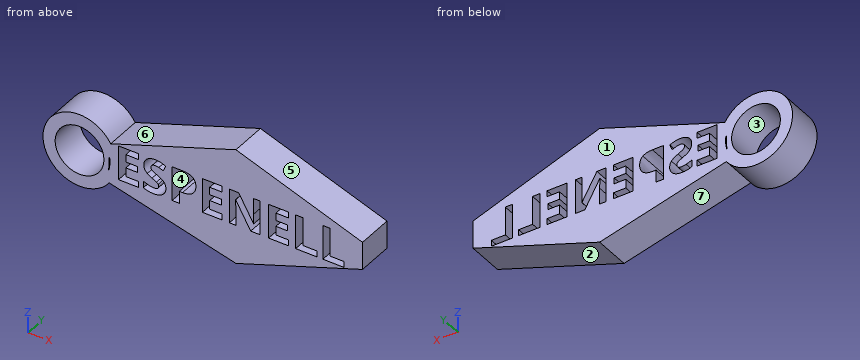
```python
from build123d import *

# Parameters (mm, degrees)
F0_R     = 10
F1_DEPTH = 15


with BuildPart() as f1:
    # F0 (on Front) → F1 (new body)
    with BuildSketch(Plane.XZ):
        with BuildLine():
            ThreePointArc((-51.9289774608, 2.6432993809), (-51.6588535234, -0.5600733653), (-52.2146643877, -3.726402182))
            Line((-52.2146643877, -3.726402182), (-52.2146643877, -8.726402182))
            Line((-52.2146643877, -8.726402182), (-51.9870151319, -8.7836093454))
            ThreePointArc((-51.9870151319, -8.7836093454), (-49.874136957, -4.6157733907), (-49.1462999327, 0))
            ThreePointArc((-49.1462999327, 0), (-49.7101962212, 4.0741759452), (-51.3594878837, 7.8420301978))
            Line((-51.3594878837, 7.8420301978), (-51.9289774608, 7.6432993809))
            Line((-51.9289774608, 7.6432993809), (-51.9289774608, 2.6432993809))
        make_face()
        with BuildLine():
            Line((-52.2146643877, -8.726402182), (-52.2146643877, -3.726402182))
            Line((-52.2146643877, -3.726402182), (-51.9289774608, 2.6432993809))
            Line((-51.9289774608, 2.6432993809), (-51.9289774608, 7.6432993809))
            Line((-51.9289774608, 7.6432993809), (-51.3594878837, 7.8420301978))
            ThreePointArc((-51.3594878837, 7.8420301978), (-79.1356264541, 0.565765353), (-51.9870151319, -8.7836093454))
            Line((-51.9870151319, -8.7836093454), (-52.2146643877, -8.726402182))
        make_face()
        with Locations((-64.1462999327, 0)):
            Circle(F0_R, mode=Mode.SUBTRACT)
        with BuildLine():
            ThreePointArc((-49.1462999327, 0), (-49.874136957, -4.6157733907), (-51.9870151319, -8.7836093454))
            Line((-51.9870151319, -8.7836093454), (0, -21.8476962826))
            Line((0, -21.8476962826), (51.9289774608, -3.726402182))
            Line((51.9289774608, -3.726402182), (51.9289774608, 7.6432993809))
            Line((51.9289774608, 7.6432993809), (0, 25.7645934815))
            Line((0, 25.7645934815), (-51.3594878837, 7.8420301978))
            ThreePointArc((-51.3594878837, 7.8420301978), (-49.7101962212, 4.0741759452), (-49.1462999327, 0))
        make_face()
        Polygon((-40.0178585444, -3.4319313488), (-40.0178585444, -5.9052360061), (-48.1519392362, -5.9052360061), (-48.1519392362, 8.2204252181), (-40.0178585444, 8.2204252181), (-40.0178585444, 5.7656703457), (-45.15614897, 5.7656703457), (-45.15614897, 2.6647646316), (-40.3733960889, 2.6647646316), (-40.3733960889, 0.2100097592), (-45.15614897, 0.2100097592), (-45.15614897, -3.4319313488), align=None, mode=Mode.SUBTRACT)
        with BuildLine():
            add(Edge.make_bspline(
                [(-29.4676683654, 0.3506789616), (-28.7334060453, -0.5999975161), (-28.7334060453, -1.9819564934)],
                knots=[0, 0, 0, 1, 1, 1], degree=2))
            add(Edge.make_bspline(
                [(-28.7334060453, -1.9819564934), (-28.7334060453, -3.895675972), (-30.1107275763, -4.9978423599)],
                knots=[0, 0, 0, 1, 1, 1], degree=2))
            add(Edge.make_bspline(
                [(-30.1107275763, -4.9978423599), (-31.4880491074, -6.1000087479), (-33.939712349, -6.1000087479)],
                knots=[0, 0, 0, 1, 1, 1], degree=2))
            add(Edge.make_bspline(
                [(-33.939712349, -6.1000087479), (-36.2027861105, -6.1000087479), (-37.9402826322, -5.2467186411)],
                knots=[0, 0, 0, 1, 1, 1], degree=2))
            Line((-37.9402826322, -5.2467186411), (-37.9402826322, -2.4642509016))
            add(Edge.make_bspline(
                [(-37.9402826322, -2.4642509016), (-36.5119491926, -3.1042184817), (-35.5210815143, -3.3639154707)],
                knots=[0, 0, 0, 1, 1, 1], degree=2))
            add(Edge.make_bspline(
                [(-35.5210815143, -3.3639154707), (-34.5302138359, -3.6236124597), (-33.7078400374, -3.6236124597)],
                knots=[0, 0, 0, 1, 1, 1], degree=2))
            add(Edge.make_bspline(
                [(-33.7078400374, -3.6236124597), (-32.7247014361, -3.6236124597), (-32.197578381, -3.2479793149)],
                knots=[0, 0, 0, 1, 1, 1], degree=2))
            add(Edge.make_bspline(
                [(-32.197578381, -3.2479793149), (-31.6704553259, -2.87234617), (-31.6704553259, -2.127263142)],
                knots=[0, 0, 0, 1, 1, 1], degree=2))
            add(Edge.make_bspline(
                [(-31.6704553259, -2.127263142), (-31.6704553259, -1.7129846119), (-31.9023276375, -1.3883633756)],
                knots=[0, 0, 0, 1, 1, 1], degree=2))
            add(Edge.make_bspline(
                [(-31.9023276375, -1.3883633756), (-32.1341999491, -1.0637421394), (-32.5840322337, -0.7653997651)],
                knots=[0, 0, 0, 1, 1, 1], degree=2))
            add(Edge.make_bspline(
                [(-32.5840322337, -0.7653997651), (-33.0338645182, -0.4670573908), (-34.4158234955, 0.1914599742)],
                knots=[0, 0, 0, 1, 1, 1], degree=2))
            add(Edge.make_bspline(
                [(-34.4158234955, 0.1914599742), (-35.708125179, 0.8005112461), (-36.3558218361, 1.3600964248)],
                knots=[0, 0, 0, 1, 1, 1], degree=2))
            add(Edge.make_bspline(
                [(-36.3558218361, 1.3600964248), (-37.0035184933, 1.9196816036), (-37.389972346, 2.6647646316)],
                knots=[0, 0, 0, 1, 1, 1], degree=2))
            add(Edge.make_bspline(
                [(-37.389972346, 2.6647646316), (-37.7764261987, 3.4098476596), (-37.7764261987, 4.4022611534)],
                knots=[0, 0, 0, 1, 1, 1], degree=2))
            add(Edge.make_bspline(
                [(-37.7764261987, 4.4022611534), (-37.7764261987, 6.2788810621), (-36.505765931, 7.3501311418)],
                knots=[0, 0, 0, 1, 1, 1], degree=2))
            add(Edge.make_bspline(
                [(-36.505765931, 7.3501311418), (-35.2351056633, 8.4213812215), (-32.9936733176, 8.4213812215)],
                knots=[0, 0, 0, 1, 1, 1], degree=2))
            add(Edge.make_bspline(
                [(-32.9936733176, 8.4213812215), (-31.893052745, 8.4213812215), (-30.8929101742, 8.1616842325)],
                knots=[0, 0, 0, 1, 1, 1], degree=2))
            add(Edge.make_bspline(
                [(-30.8929101742, 8.1616842325), (-29.8927676034, 7.9019872435), (-28.8014219234, 7.4289677278)],
                knots=[0, 0, 0, 1, 1, 1], degree=2))
            Line((-28.8014219234, 7.4289677278), (-29.7660107397, 5.0978780882))
            add(Edge.make_bspline(
                [(-29.7660107397, 5.0978780882), (-30.8975476205, 5.5616227115), (-31.6364473868, 5.7455747454)],
                knots=[0, 0, 0, 1, 1, 1], degree=2))
            add(Edge.make_bspline(
                [(-31.6364473868, 5.7455747454), (-32.3753471532, 5.9295267793), (-33.089513873, 5.9295267793)],
                knots=[0, 0, 0, 1, 1, 1], degree=2))
            add(Edge.make_bspline(
                [(-33.089513873, 5.9295267793), (-33.939712349, 5.9295267793), (-34.3941820798, 5.5337980341)],
                knots=[0, 0, 0, 1, 1, 1], degree=2))
            add(Edge.make_bspline(
                [(-34.3941820798, 5.5337980341), (-34.8486518106, 5.1380692889), (-34.8486518106, 4.5011933396)],
                knots=[0, 0, 0, 1, 1, 1], degree=2))
            add(Edge.make_bspline(
                [(-34.8486518106, 4.5011933396), (-34.8486518106, 4.1054645945), (-34.6646997767, 3.810213851)],
                knots=[0, 0, 0, 1, 1, 1], degree=2))
            add(Edge.make_bspline(
                [(-34.6646997767, 3.810213851), (-34.4807477428, 3.5149631075), (-34.0803815514, 3.2398079644)],
                knots=[0, 0, 0, 1, 1, 1], degree=2))
            add(Edge.make_bspline(
                [(-34.0803815514, 3.2398079644), (-33.68001536, 2.9646528213), (-32.1836660423, 2.2504861015)],
                knots=[0, 0, 0, 1, 1, 1], degree=2))
            add(Edge.make_bspline(
                [(-32.1836660423, 2.2504861015), (-30.2019306856, 1.3013554392), (-29.4676683654, 0.3506789616)],
                knots=[0, 0, 0, 1, 1, 1], degree=2))
        make_face(mode=Mode.SUBTRACT)
        with BuildLine():
            add(Edge.make_bspline(
                [(-17.7534791821, 7.113621384), (-16.4163488518, 6.0068175498), (-16.4163488518, 3.8148512972)],
                knots=[0, 0, 0, 1, 1, 1], degree=2))
            add(Edge.make_bspline(
                [(-16.4163488518, 3.8148512972), (-16.4163488518, 1.5332277508), (-17.8415906605, 0.325945915)],
                knots=[0, 0, 0, 1, 1, 1], degree=2))
            add(Edge.make_bspline(
                [(-17.8415906605, 0.325945915), (-19.2668324693, -0.8813359209), (-21.8947186678, -0.8813359209)],
                knots=[0, 0, 0, 1, 1, 1], degree=2))
            Line((-21.8947186678, -0.8813359209), (-23.1777454587, -0.8813359209))
            Line((-23.1777454587, -0.8813359209), (-23.1777454587, -5.9052360061))
            Line((-23.1777454587, -5.9052360061), (-26.1735357249, -5.9052360061))
            Line((-26.1735357249, -5.9052360061), (-26.1735357249, 8.2204252181))
            Line((-26.1735357249, 8.2204252181), (-21.6628463561, 8.2204252181))
            add(Edge.make_bspline(
                [(-21.6628463561, 8.2204252181), (-19.0906095125, 8.2204252181), (-17.7534791821, 7.113621384)],
                knots=[0, 0, 0, 1, 1, 1], degree=2))
        make_face(mode=Mode.SUBTRACT)
        Polygon((-5.6141907608, -3.4319313488), (-5.6141907608, -5.9052360061), (-13.7482714526, -5.9052360061), (-13.7482714526, 8.2204252181), (-5.6141907608, 8.2204252181), (-5.6141907608, 5.7656703457), (-10.7524811864, 5.7656703457), (-10.7524811864, 2.6647646316), (-5.9697283053, 2.6647646316), (-5.9697283053, 0.2100097592), (-10.7524811864, 0.2100097592), (-10.7524811864, -3.4319313488), align=None, mode=Mode.SUBTRACT)
        with BuildLine():
            Line((9.8625131325, 8.2204252181), (9.8625131325, -5.9052360061))
            Line((9.8625131325, -5.9052360061), (6.056715591, -5.9052360061))
            Line((6.056715591, -5.9052360061), (-0.0894464825, 4.7794401136))
            Line((-0.0894464825, 4.7794401136), (-0.1760121455, 4.7794401136))
            add(Edge.make_bspline(
                [(-0.1760121455, 4.7794401136), (0.0094857038, 1.9505979118), (0.0094857038, 0.7417702605)],
                knots=[0, 0, 0, 1, 1, 1], degree=2))
            Line((0.0094857038, 0.7417702605), (0.0094857038, -5.9052360061))
            Line((0.0094857038, -5.9052360061), (-2.6678665878, -5.9052360061))
            Line((-2.6678665878, -5.9052360061), (-2.6678665878, 8.2204252181))
            Line((-2.6678665878, 8.2204252181), (1.1101062763, 8.2204252181))
            Line((1.1101062763, 8.2204252181), (7.2439018265, -2.3591354536))
            Line((7.2439018265, -2.3591354536), (7.3119177046, -2.3591354536))
            add(Edge.make_bspline(
                [(7.3119177046, -2.3591354536), (7.166611056, 0.3955076085), (7.166611056, 1.5332277508)],
                knots=[0, 0, 0, 1, 1, 1], degree=2))
            Line((7.166611056, 1.5332277508), (7.166611056, 8.2204252181))
            Line((7.166611056, 8.2204252181), (9.8625131325, 8.2204252181))
        make_face(mode=Mode.SUBTRACT)
        Polygon((21.5519692692, -3.4319313488), (21.5519692692, -5.9052360061), (13.4178885774, -5.9052360061), (13.4178885774, 8.2204252181), (21.5519692692, 8.2204252181), (21.5519692692, 5.7656703457), (16.4136788436, 5.7656703457), (16.4136788436, 2.6647646316), (21.1964317247, 2.6647646316), (21.1964317247, 0.2100097592), (16.4136788436, 0.2100097592), (16.4136788436, -3.4319313488), align=None, mode=Mode.SUBTRACT)
        Polygon((33.222875621, -5.9052360061), (24.4982934423, -5.9052360061), (24.4982934423, 8.2204252181), (27.4940837085, 8.2204252181), (27.4940837085, -3.4319313488), (33.222875621, -3.4319313488), align=None, mode=Mode.SUBTRACT)
        Polygon((44.4022126722, -5.9052360061), (35.6776304934, -5.9052360061), (35.6776304934, 8.2204252181), (38.6734207596, 8.2204252181), (38.6734207596, -3.4319313488), (44.4022126722, -3.4319313488), align=None, mode=Mode.SUBTRACT)
    extrude(amount=F1_DEPTH)


solid = f1.part
```
Geometry check sheet. Reference: the model listing, model coordinates, mm. Face numbers are marked on the shaded views. A direction names the side the tool comes from. Give positions to 0.01 mm unless a question says otherwise; leave off trailing zeros. Write each loop counter-clockwise with the first axis right and the second up, starting at its lowest first coordinate (ties: lowest second). Pieces come first, ordered by that corner, then holes.
1) Section check D-D, the plane y = -1.5. State how many separate pieces and enclosed holes the cut face has, and give its area (3 significant figures).
2) Material ranges on L1, parallel to Z at x = 31.5, y = -3.25; L2, parallel to Z at x = 16.5, y = -2.25; L3, parallel to Z at x = 30, y = -10.25, recorded low to high.
3) Access from +Z, -Z, +X, -X, +Y, -Y to the whole of each face (thin tool, end or side, straight path). Record for the marked faces 4, 5, 6 and 7.
4) Section check A-A, the plane z = -7.5. Record the boundary of the cut face in (x, y), and give its area (3 significant figures).
5) Gauge pin test, flat ends, axial feed: pin 1 (8 mm diameter, centred on x = -49, z = -16.5, fed in from -Y); pin 2 (2.5 mm diameter, centred on y = -7.5, z = -5, fed in from -X); pin 3 (2.5 mm diameter, centred on x = 18, y = -7.5, fed in from +Z); pin 4 (2 mm diameter, centred on x = 38, y = -1.5, fed in from -Z). Record the tip position at first contact, or that the pin passes through.
6) Release check for a two-part mould opening along X. For the marked faces 1, 2 and 3 record: pulls with the +X half, pulls with the -X half, needs draft (parallel to the pull), parting line crosses it, or undercut.
7) Section check C-C, the plane x = -8. Record the boundary of the cut face in (y, z), and give its area (3 significant figures).
8) Section check B-B, the plane x = -60. Record the boundary of the cut face in (y, z).
Computed:
1. separate pieces: 1
1. enclosed holes: 10
1. area: 2,920 mm2
2. L1: z = -10.86 to -5.91, -3.43 to 14.77
2. L2: z = -16.09 to -5.91, -3.43 to 0.21, 2.66 to 5.77, 8.22 to 20.01
2. L3: z = -11.38 to -5.91, -3.43 to 15.3
3. face 4: +Y, -Y
3. face 5: +Z, +X, +Y, -Y
3. face 6: +Z, +Y, -Y
3. face 7: -Z, +Y, -Y
4. outline: (-77.14, -15) - (-70.76, -15) - (-70.76, 0) - (-77.14, 0) - close; (-57.53, -15) - (41.12, -15) - (41.12, 0) - (-57.53, 0) - close
4. area: 1,580 mm2
5. pin 1: passes through
5. pin 2: stops at x = -78.67
5. pin 3: stops at z = 19.92
5. pin 4: stops at z = -8.94
6. face 1: needs draft
6. face 2: pulls with the +X half
6. face 3: undercut
7. outline: (-15, -19.84) - (0, -19.84) - (0, -5.91) - (-15, -5.91) - close; (-15, -3.43) - (0, -3.43) - (0, 0.21) - (-15, 0.21) - close; (-15, 2.66) - (0, 2.66) - (0, 5.77) - (-15, 5.77) - close; (-15, 8.22) - (0, 8.22) - (0, 22.97) - (-15, 22.97) - close
7. area: 531 mm2
8. outline: (-15, -14.42) - (0, -14.42) - (0, -9.1) - (-15, -9.1) - close; (-15, 9.1) - (0, 9.1) - (0, 14.42) - (-15, 14.42) - close
